Geometry check sheet. Reference: drawing and pictorial views, mm from the part's lowest x, y, z. A direction names the side the tool comes from. Round coordinates to 2 decimals unless told otherwise and drop trailing zeros. Order: outer loops, then holes, each group sorted by start corner. A loop starts at its lowest first (then second) coordinate and runs counter-clockwise, first axis right, second up. Notation, with made-up numbers: M 46.25,32.25 L 75.25,32.25 A8 ccw 75.25,44.25 Z; hole C -38,47.25 d8. An arc over 180 degrees is marked long. Answer as a JSON object with one key per item and string values. Group by question number.
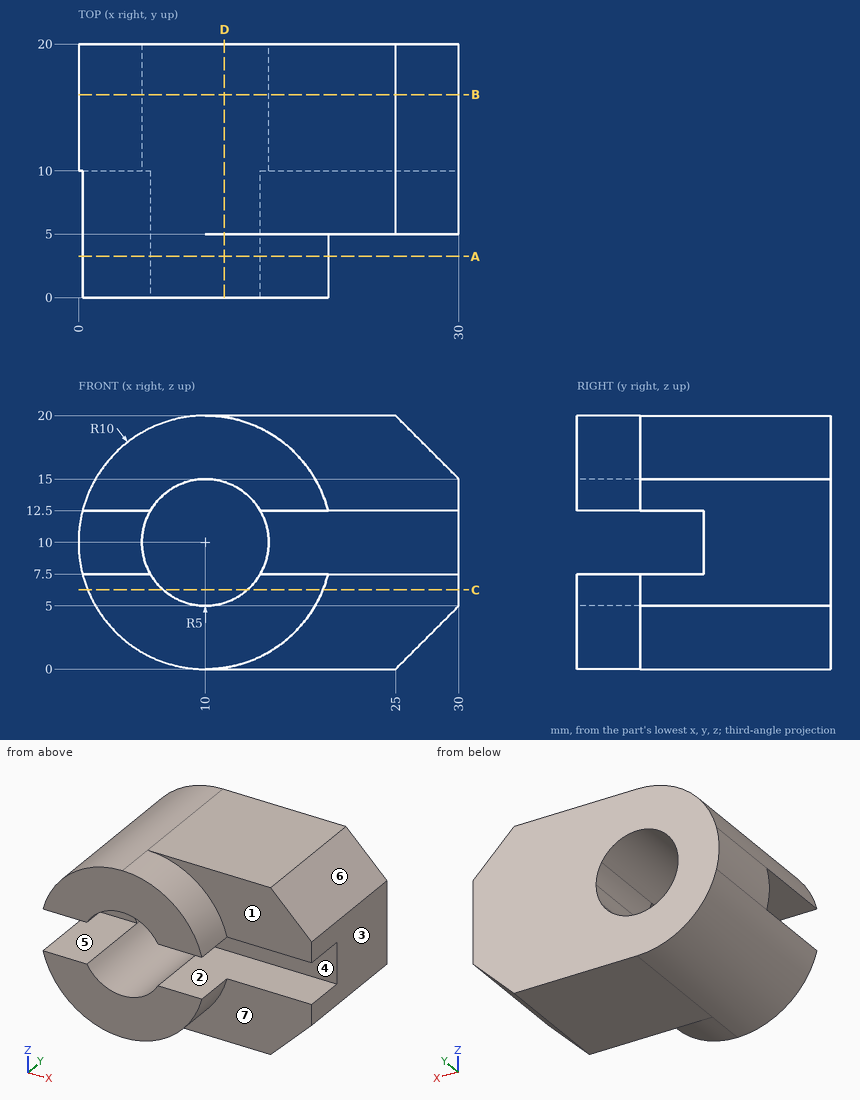
Q1. Tool access check on the marked faces 1, 2 and 3. Record the directions out of +Z, -Z, +X, -X, +Y, -Y that give a thin tool (end or side, any length) a straight path to the whole face; none if there is none.
Q2. Release check for a two-part mould opening along Z. For the marked faces 4, 5, 6 and 7 record: released by +Z, released by -Z, zero draft, split by the parting line, or undercut.
Q3. Cross-section at D-D, the plane x = 11.5. Record the cut outline in (y, z).
Q4. Gauge pin test, flat ends, axial feed: pin 1 Ø5 at (y, z) = (7.5, 6.5) entering from -X; pin 2 Ø1.5 at (x, y) = (6.5, 7) entering from -Z; pin 3 Ø4 at (x, z) = (24.5, 3.5) entering from -Y; pin 4 Ø4 at (y, z) = (5.5, 10) entering from +X. Record the tip position at first contact, or that the pin passes through.
Q5. Cross-section at C-C, the plane z = 6.25. Record the cut outline in (x, y).
Q6. Cross-section at A-A, the plane y = 3.25. Record the cut outline in (x, z).
Q7. Cross-section at B-B, the plane y = 16. Record the cut outline in (x, z).
Q8. Thickness scan on line 1 (Z direction, x = 10, y = 3.5); line 2 (X direction, y = 17, z = 7.5); line 3 (Z direction, x = 24.25, y = 5.25). Record the ranges inside material, lowest first. Write a range as from..to.
Conclusion:
{
 "1": {"face 1": "+Z, +X, -Y", "face 2": "+X, -X, -Y", "face 3": "+Z, -Z, +X, +Y, -Y"},
 "2": {"face 4": "undercut", "face 5": "undercut", "face 6": "released by +Z", "face 7": "zero draft"},
 "3": {"outline": "M 0,0.11 L 5,0.11 L 5,0 L 20,0 L 20,5.23 L 0,5.23 Z; M 0,14.77 L 20,14.77 L 20,20 L 5,20 L 5,19.89 L 0,19.89 Z"},
 "4": {"pin 1": "x = 0.32", "pin 2": "z = 0.39", "pin 3": "y = 5", "pin 4": "through"},
 "5": {"outline": "M 0.73,0 L 6.69,0 L 6.69,20 L 0.73,20 Z; M 13.31,0 L 19.27,0 L 19.27,5 L 30,5 L 30,20 L 13.31,20 Z"},
 "6": {"outline": "M 0.32,7.5 A10 ccw 10,0 A10 ccw 19.68,7.5 L 14.33,7.5 A5 cw 5.67,7.5 Z; M 0.32,12.5 L 5.67,12.5 A5 cw 14.33,12.5 L 19.68,12.5 A10 ccw 10,20 A10 ccw Z"},
 "7": {"outline": "M 0.32,7.5 A10 ccw 10,0 L 25,0 L 30,5 L 30,15 L 25,20 L 10,20 A10 ccw 0.32,12.5 A10 ccw Z; hole M 14.33,7.5 A5 ccw 15,10 A5 ccw 14.33,12.5 A5 ccw long Z"},
 "8": {"line 1": "0..5, 15..20", "line 2": "0.32..5.67, 14.33..30", "line 3": "0..7.5, 12.5..20"}
}
